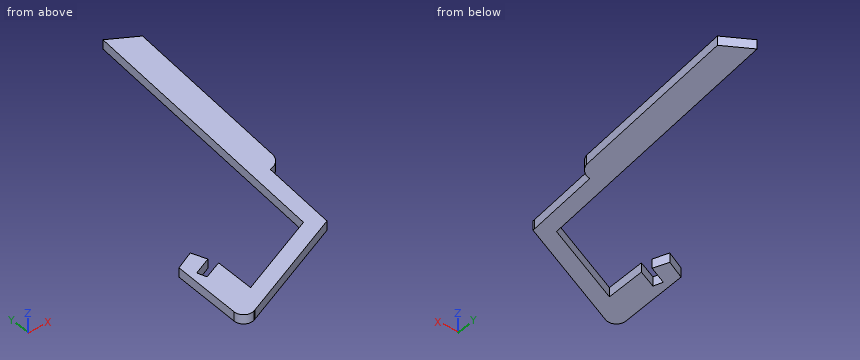
from build123d import *

# Parameters (mm, degrees)
BASE_EXTRUDE_DEPTH = 3


with BuildPart() as part:
    # Sketch1 → Base-Extrude (new body)
    with BuildSketch(Plane.XY):
        with BuildLine():
            Line((827.973978263, -43.245786047), (829.514372586, -18.937919224))
            ThreePointArc((829.514372586, -18.937919224), (832.162066859, -17.653066314), (833.626640717, -15.100390193))
            Line((833.626640717, -15.100390193), (837.267672807, 42.356146641))
            Line((837.267672807, 42.356146641), (828.567150472, 47.366870762))
            Line((828.567150472, 47.366870762), (822.996025927, -40.547081848))
            Line((822.996025927, -40.547081848), (796.525541864, -52.540147354))
            Line((796.525541864, -52.540147354), (796.34247294, -39.8809937))
            Line((796.34247294, -39.8809937), (790.624612073, -42.415731004))
            Line((790.624612073, -42.415731004), (789.560278608, -39.610879088))
            Line((789.560278608, -39.610879088), (795.188053447, -37.002397586))
            Line((795.188053447, -37.002397586), (793.171716746, -32.401991353))
            Line((793.171716746, -32.401991353), (787.326904418, -35.230416068))
            Line((787.326904418, -35.230416068), (787.326904418, -57.526741279))
            ThreePointArc((787.326904418, -57.526741279), (788.61109588, -59.98763564), (791.364238458, -60.341690318))
            ThreePointArc((791.364238458, -60.341690318), (791.701286321, -60.210514776), (792.033370234, -60.067236869))
            Line((792.033370234, -60.067236869), (827.968278958, -43.7860947))
            ThreePointArc((827.968278958, -43.7860947), (827.974778648, -43.515978875), (827.973978263, -43.245786047))
        make_face()
    extrude(amount=BASE_EXTRUDE_DEPTH)


solid = part.part
Read the model definition and answer for the solid it produces. Units are mm, in the model's axes. Give positions to 0.01 mm unless a question says otherwise; leave off trailing zeros. Write each loop counter-clockwise with the first axis right and the second up, starting at its lowest first coordinate (ties: lowest second). Pieces come first, ordered by that corner, then holes. Notation, with made-up numbers: (80.25, -29) -> (111.25, -29) arc R19 ccw to (111.25, -4) -> close; hole circle Ø10 at (39, 52.25). An arc over 180 degrees is marked (long way). Answer as a JSON object with one key per item and string values. Group by question number.
1) Consider L1, parallel to Y at x = 795, z = 0.3; L2, parallel to X at y = -42, z = 2.65; L3, parallel to X at y = 16, z = 0.4. Determine where each line is inside the solid, lowest interval first. Write a range as from..to.
2) Find section D-D (y = 9). Write down the section's boundary in (x, z), and give its area (3 significant figures).
3) Find section A-A (z = 2.5). Write down the section's boundary in (x, y), and give its area (3 significant figures).
4) Find section C-C (x = 818). Write down the section's boundary in (y, z), and give its area (3 significant figures).
5) Each of these flat-tipped pins is pushed along its axis until it touches: P1, Ø8, axis at x = 826, y = 18.5, coming from the -Z side; P2, Ø4, axis at x = 803, y = -46, coming from the +Z side; P3, Ø1.5, axis at y = -44, z = 0.5, coming from the +X side. Where does it stop, or does it pass through?
6) Find section B-B (y = -38.5). Write down the section's boundary in (x, z).
Values follow:
{
 "1": {"L1": "y = -58.72..-40.48, -37.09..-36.57", "L2": "x = 787.33..790.47, 791.56..796.37, 819.79..828.05", "L3": "x = 826.58..835.6"},
 "2": {"outline": "(826.14, 0) -> (835.15, 0) -> (835.15, 3) -> (826.14, 3) -> close", "area": "27.1 mm2"},
 "3": {"outline": "(787.33, -57.53) arc R3 ccw to (791.36, -60.34) arc R10 ccw to (792.03, -60.07) -> (827.97, -43.79) arc R10 ccw to (827.97, -43.25) -> (829.51, -18.94) arc R4.99 ccw to (833.63, -15.1) -> (837.27, 42.36) -> (828.57, 47.37) -> (823, -40.55) -> (796.53, -52.54) -> (796.34, -39.88) -> (790.62, -42.42) -> (789.56, -39.61) -> (795.19, -37) -> (793.17, -32.4) -> (787.33, -35.23) -> close", "area": "1,060 mm2"},
 "4": {"outline": "(-48.3, 0) -> (-42.81, 0) -> (-42.81, 3) -> (-48.3, 3) -> close", "area": "16.5 mm2"},
 "5": {"P1": "stops at z = 0", "P2": "passes through", "P3": "stops at x = 827.98"},
 "6": {"outline": "(787.33, 0) -> (791.96, 0) -> (791.96, 3) -> (787.33, 3) -> close; (823.13, 0) -> (828.27, 0) -> (828.27, 3) -> (823.13, 3) -> close"}
}
